Verification items for the finished model (mm, model axes). Coordinates: 2 decimals unless noted, no trailing zeros. Order: outer loops, then holes, each group sorted by start corner. A loop starts at its lowest first (then second) coordinate and runs counter-clockwise, first axis right, second up. Notation, with made-up numbers: M 29,35 L 57,35 A34 ccw 57,67 Z; hole C 29.25,68.25 d5. An arc over 180 degrees is marked long. Return JSON: item names as keys, results as strings. Group by question number.
1. Material ranges on line 1 along Y through (x, z) = (6, 0.95); line 2 along Y through (x, z) = (0, 1.65); line 3 along X through (y, z) = (-4, 2.15), recorded low to high.
2. Section check B-B, the plane x = -12. Record the cut outline in (y, z).
3. Section check A-A, the plane z = 1.1. Record the cut outline in (x, y), plus the area to 3 significant figures.
4. Mould release check, pull along Y, two halves, no side actions. Record for faces 1 (the flat face through (0, -10, 1)), 2 (the cylindrical face through (-0.17, 4.29, 1.38)), 3 (the flat face through (0, 0, 3)), 4 (the cylindrical face through (13.24, -2.61, 1.38)): +Y half, -Y half, draft (parallel to the pull), parting line (faces both ways), or undercut.
5. Section check C-C, the plane y = -3.5. Give the number of separate pieces and of enclosed holes in the cut face, plus the area to 3 significant figures.
6. Gauge pin test, flat end, axial feed: pin 1 (1.6 mm diameter, centred on x = 6, y = -3, fed in from +Z). Record the tip position at first contact, or that the pin passes through.
```python
from build123d import *

# Parameters (mm, degrees)
SKETCH_1_W      = 34
SKETCH_1_H      = 20
SKETCH_1_R      = 1.3
EXTRUDE_1_DEPTH = 3
CHAMFER_1_SIZE  = 0.2


with BuildPart() as part:
    # 草圖1 → 填料-伸長1 (new body)
    with BuildSketch(Plane.XY):
        Rectangle(SKETCH_1_W, SKETCH_1_H)
        with Locations((0, 3)):
            Circle(SKETCH_1_R, mode=Mode.SUBTRACT)
        with Locations((-6, -3)):
            Circle(SKETCH_1_R, mode=Mode.SUBTRACT)
        with Locations((6, -3)):
            Circle(SKETCH_1_R, mode=Mode.SUBTRACT)
        with Locations((12, -3)):
            Circle(SKETCH_1_R, mode=Mode.SUBTRACT)
        with Locations((-12, -3)):
            Circle(SKETCH_1_R, mode=Mode.SUBTRACT)
    extrude(amount=EXTRUDE_1_DEPTH)

    # 導角1
    chamfer_1_edges = [part.edges().sort_by_distance(p)[0] for p in [
        (-13.3, -3, 3),
        (-1.3, 3, 3),
        (4.7, -3, 3),
        (-7.3, -3, 3),
        (10.7, -3, 3),
    ]]
    chamfer(chamfer_1_edges, length=CHAMFER_1_SIZE)


solid = part.part
```
Answers follow:
{
 "1": {"line 1": "-10 to -4.3, -1.7 to 10", "line 2": "-10 to 1.7, 4.3 to 10", "line 3": "-17 to -12.83, -11.17 to -6.83, -5.17 to 5.17, 6.83 to 11.17, 12.83 to 17"},
 "2": {"outline": "M -10,0 L -4.3,0 L -4.3,2.8 L -4.5,3 L -10,3 Z; M -1.7,0 L 10,0 L 10,3 L -1.5,3 L -1.7,2.8 Z"},
 "3": {"outline": "M -17,-10 L 17,-10 L 17,10 L -17,10 Z; hole C -12,-3 d2.6; hole C -6,-3 d2.6; hole C 0,3 d2.6; hole C 6,-3 d2.6; hole C 12,-3 d2.6", "area": "653 mm^2"},
 "4": {"face 1": "-Y half", "face 2": "undercut", "face 3": "draft", "face 4": "undercut"},
 "5": {"separate pieces": "5", "enclosed holes": "0", "area": "73.0 mm^2"},
 "6": {"pin 1": "through"}
}
